from build123d import *

# Parameters (mm, degrees)
BOSS_EXTRUDE3_DEPTH     = 35
CUT_EXTRUDE4_START      = -33
CUT_EXTRUDE4_DEPTH      = 33
SHELL3_DEPTH            = 33
BOSS_EXTRUDE5_START     = 1
BOSS_EXTRUDE5_DEPTH     = 1
CUT_EXTRUDE5_DEPTH      = 88.114866699
CUT_EXTRUDE5_DEPTH_BACK = 88.114866699
SKETCH10_R              = 1.5
FILLET6_R               = 2
FILLET8_R               = 2
CUT_EXTRUDE7_REACH      = 151.75
SKETCH13_W              = 20
SKETCH13_H              = 20
CUT_EXTRUDE10_REACH     = 113.915
SKETCH16_W              = 19.05
SKETCH16_H              = 12.7
FILLET11_R              = 1


# Read off the part's stored shape, not the designer's step: Shell3
with BuildPart() as part:
    # Sketch4 → Boss-Extrude3 (new body)
    with BuildSketch(Plane(origin=(0, 0, 0), x_dir=(1, 0, 0), z_dir=(0, 1, 0))):
        with BuildLine():
            Line((-63, 40), (63, 40))
            ThreePointArc((63, 40), (67.949747468, 37.949747468), (70, 33))
            Line((70, 33), (70, -33))
            ThreePointArc((70, -33), (67.949747468, -37.949747468), (63, -40))
            Line((63, -40), (-63, -40))
            ThreePointArc((-63, -40), (-67.949747468, -37.949747468), (-70, -33))
            Line((-70, -33), (-70, 33))
            ThreePointArc((-70, 33), (-67.949747468, 37.949747468), (-63, 40))
        make_face()
    extrude(amount=BOSS_EXTRUDE3_DEPTH)

    # Sketch9 → Cut-Extrude4 (cut)
    with BuildSketch(Plane(origin=(0, 35, 0), x_dir=(1, 0, 0), z_dir=(0, 1, 0)).offset(CUT_EXTRUDE4_START)):
        with BuildLine():
            Line((-63, 26), (-70, 26))
            Line((-70, 26), (-70, 33))
            ThreePointArc((-70, 33), (-67.949747468, 37.949747468), (-63, 40))
            Line((-63, 40), (-56, 40))
            Line((-56, 40), (-56, 33))
            ThreePointArc((-56, 33), (-58.050252532, 28.050252532), (-63, 26))
        make_face()
        with BuildLine():
            Line((-63, -26), (-70, -26))
            Line((-70, -26), (-70, -33))
            ThreePointArc((-70, -33), (-67.949747468, -37.949747468), (-63, -40))
            Line((-63, -40), (-56, -40))
            Line((-56, -40), (-56, -33))
            ThreePointArc((-56, -33), (-58.050252532, -28.050252532), (-63, -26))
        make_face()
        with BuildLine():
            Line((56, -33), (56, -40))
            Line((56, -40), (63, -40))
            ThreePointArc((63, -40), (67.949747468, -37.949747468), (70, -33))
            Line((70, -33), (70, -26))
            Line((70, -26), (63, -26))
            ThreePointArc((63, -26), (58.050252532, -28.050252532), (56, -33))
        make_face()
        with BuildLine():
            Line((56, 33), (56, 40))
            Line((56, 40), (63, 40))
            ThreePointArc((63, 40), (67.949747468, 37.949747468), (70, 33))
            Line((70, 33), (70, 26))
            Line((70, 26), (63, 26))
            ThreePointArc((63, 26), (58.050252532, 28.050252532), (56, 33))
        make_face()
    extrude(amount=CUT_EXTRUDE4_DEPTH, mode=Mode.SUBTRACT)

    # Shell3 outline → Shell3 (cut)
    with BuildSketch(Plane(origin=(0, 0, 0), x_dir=(1, 0, 0), z_dir=(0, 1, 0))):
        with BuildLine():
            Line((-68, 24), (-68, -25.516685226))
            ThreePointArc((-68, -25.516685226), (-56.636038969, -26.636038969), (-55.516685226, -38))
            Line((-55.516685226, -38), (55.516685226, -38))
            ThreePointArc((55.516685226, -38), (56.636038969, -26.636038969), (68, -25.516685226))
            Line((68, -25.516685226), (68, 24))
            Line((68, 24), (63, 24))
            ThreePointArc((63, 24), (56.636038969, 26.636038969), (54, 33))
            Line((54, 33), (54, 38))
            Line((54, 38), (-54, 38))
            Line((-54, 38), (-54, 33))
            ThreePointArc((-54, 33), (-56.636038969, 26.636038969), (-63, 24))
            Line((-63, 24), (-68, 24))
        make_face()
    extrude(amount=SHELL3_DEPTH, mode=Mode.SUBTRACT)

    # Sketch11 → Boss-Extrude5 (add)
    with BuildSketch(Plane.XZ.offset(-1).offset(BOSS_EXTRUDE5_START)):
        with BuildLine():
            Line((68, 24), (63, 24))
            ThreePointArc((63, 24), (56.636038969, 26.636038969), (54, 33))
            Line((54, 33), (54, 38))
            Line((54, 38), (63, 38))
            ThreePointArc((63, 38), (66.535533906, 36.535533906), (68, 33))
            Line((68, 33), (68, 24))
        make_face()
        with BuildLine():
            Line((54, -33), (54, -38))
            Line((54, -38), (63, -38))
            ThreePointArc((63, -38), (66.535533906, -36.535533906), (68, -33))
            Line((68, -33), (68, -24))
            Line((68, -24), (63, -24))
            ThreePointArc((63, -24), (56.636038969, -26.636038969), (54, -33))
        make_face()
        with BuildLine():
            Line((-63, -24), (-68, -24))
            Line((-68, -24), (-68, -33))
            ThreePointArc((-68, -33), (-66.535533906, -36.535533906), (-63, -38))
            Line((-63, -38), (-54, -38))
            Line((-54, -38), (-54, -33))
            ThreePointArc((-54, -33), (-56.636038969, -26.636038969), (-63, -24))
        make_face()
        with BuildLine():
            Line((-54, 33), (-54, 38))
            Line((-54, 38), (-63, 38))
            ThreePointArc((-63, 38), (-66.535533906, 36.535533906), (-68, 33))
            Line((-68, 33), (-68, 24))
            Line((-68, 24), (-63, 24))
            ThreePointArc((-63, 24), (-56.636038969, 26.636038969), (-54, 33))
        make_face()
    extrude(amount=-BOSS_EXTRUDE5_DEPTH)

    # Sketch10 → Cut-Extrude5 (cut, two sides: drawn at the far end of the back side and taken through both)
    with BuildSketch(Plane(origin=(0, 2, 0), x_dir=(1, 0, 0), z_dir=(0, 1, 0)).offset(-CUT_EXTRUDE5_DEPTH_BACK)):
        with Locations(Location((-63, 33, 0), (0, 0, 270))):
            Circle(SKETCH10_R)
        with Locations(Location((63, 33, 0), (0, 0, 270))):
            Circle(SKETCH10_R)
        with Locations(Location((63, -33, 0), (0, 0, 270))):
            Circle(SKETCH10_R)
        with Locations(Location((-63, -33, 0), (0, 0, 270))):
            Circle(SKETCH10_R)
    extrude(amount=CUT_EXTRUDE5_DEPTH + CUT_EXTRUDE5_DEPTH_BACK, mode=Mode.SUBTRACT)

    # Fillet6
    fillet6_edges = [part.edges().sort_by_distance(p)[0] for p in [
        (68, 16.5, -24),
        (-54, 16.5, -38),
        (0, 33, -38),
        (-68, 33, 0.758342613),
        (0, 33, 38),
        (68, 33, 0.758342613),
        (-56.636038969, 33, 26.636038969),
        (-56.636038969, 33, -26.636038969),
        (-68, 16.5, -24),
        (-65.5, 33, -24),
        (-54, 33, -35.5),
        (56.636038969, 33, 26.636038969),
        (56.636038969, 33, -26.636038969),
        (54, 16.5, -38),
        (54, 33, -35.5),
        (65.5, 33, -24),
    ]]
    fillet(fillet6_edges, radius=FILLET6_R)

    # Fillet8
    fillet8_edges = [part.edges().sort_by_distance(p)[0] for p in [
        (0, 35, 40),
        (-58.050252532, 35, 28.050252532),
        (-66.5, 35, 26),
        (-56, 35, 36.5),
        (-58.050252532, 2, 28.050252532),
        (-56, 2, 36.5),
        (-66.5, 2, 26),
        (-70, 35, 0),
        (-58.050252532, 35, -28.050252532),
        (-56, 35, -36.5),
        (-66.5, 35, -26),
        (-58.050252532, 2, -28.050252532),
        (-66.5, 2, -26),
        (-56, 2, -36.5),
        (70, 35, 0),
        (58.050252532, 35, 28.050252532),
        (56, 35, 36.5),
        (66.5, 35, 26),
        (58.050252532, 2, 28.050252532),
        (66.5, 2, 26),
        (56, 2, 36.5),
        (0, 35, -40),
        (58.050252532, 35, -28.050252532),
        (66.5, 35, -26),
        (56, 35, -36.5),
        (58.050252532, 2, -28.050252532),
        (56, 2, -36.5),
        (66.5, 2, -26),
    ]]
    fillet(fillet8_edges, radius=FILLET8_R)

    # Sketch13 → Cut-Extrude7 (cut, up to next)
    with BuildSketch(Plane(origin=(70, 0, 0), x_dir=(0, 0, -1), z_dir=(1, 0, 0)), mode=Mode.PRIVATE) as cut_extrude7_sk1:
        with Locations((7.25040296, 18.065666935)):
            Rectangle(SKETCH13_W, SKETCH13_H)
    cut_extrude7_tool1 = extrude(cut_extrude7_sk1.sketch, amount=-CUT_EXTRUDE7_REACH, mode=Mode.PRIVATE) & part.part
    add(cut_extrude7_tool1.solids().sort_by_distance((70, 18.065667, -7.250403))[0], mode=Mode.SUBTRACT)

    # Sketch16 → Cut-Extrude10 (cut, up to next)
    with BuildSketch(Plane.XY.offset(40), mode=Mode.PRIVATE) as cut_extrude10_sk1:
        with Locations((-28.725, 14)):
            Rectangle(SKETCH16_W, SKETCH16_H)
    cut_extrude10_tool1 = extrude(cut_extrude10_sk1.sketch, amount=-CUT_EXTRUDE10_REACH, mode=Mode.PRIVATE) & part.part
    add(cut_extrude10_tool1.solids().sort_by_distance((-28.725, 14, 40))[0], mode=Mode.SUBTRACT)

    # Fillet11
    fillet11_edges = [part.edges().sort_by_distance(p)[0] for p in [
        (-19.2, 20.35, 39),
        (-19.2, 7.65, 39),
        (-38.25, 7.65, 39),
        (-38.25, 20.35, 39),
    ]]
    fillet(fillet11_edges, radius=FILLET11_R)


solid = part.part
Verification items for the finished model (mm, model axes). A direction names the side the tool comes from. Coordinates: 2 decimals unless noted, no trailing zeros. Order: outer loops, then holes, each group sorted by start corner. A loop starts at its lowest first (then second) coordinate and runs counter-clockwise, first axis right, second up. Notation, with made-up numbers: M 33.5,-18 L 49.5,-18 A27 ccw 49.5,9 Z; hole C -39,-10.5 d5. An arc over 180 degrees is marked long. Return JSON: item names as keys, results as strings.
1) Cross-section at A-A, the plane z = 14.5. Record the boundary of the cut face in (x, y).
Answer list:
{"outline": "M -70,0 L -68,0 L -68,31 A2 cw -66,33 L 66,33 A2 cw 68,31 L 68,0 L 70,0 L 70,33 A2 ccw 68,35 L -68,35 A2 ccw -70,33 Z"}
2) Gauge pin test, flat ends, axial feed: pin 1 (0.8 mm diameter, centred on x = -55, z = 35.5, fed in from +Y); pin 2 (7.5 mm diameter, centred on x = 65.5, y = 15.5, fed in from -Z); pin 3 (3.5 mm diameter, centred on y = 16.5, z = 36.5, fed in from -X); pin 4 (3.5 mm diameter, centred on x = -63, z = -33, fed in from -Y). Record the tip position at first contact, or that the pin passes through.
Answer list:
{"pin 1": "y = 34.91", "pin 2": "z = -26.11", "pin 3": "x = -56", "pin 4": "y = 0"}
3) Release check for a two-part mould opening along X. For faces 1 (the cylindrical face through (56.76, 15.283, 26.515)), 2 (the cylindrical face through (67.9, 1, -38)), 3 (the cylindrical face through (-58, 18.3, -28.1)), 4 (the flat face through (1, 16, 40)) record: +X half, -X half, draft (parallel to the pull), parting line (faces both ways), or undercut.
Answer list:
{"face 1": "undercut", "face 2": "+X half", "face 3": "-X half", "face 4": "draft"}
4) Thickness scan on L1, parallel to Z at x = 63, y = 0.7; L2, parallel to X at y = 7, z = -21.5; L3, parallel to Z at x = 15, y = 24.5. Record the ranges inside material, lowest first. Write a range as [from, to].
Answer list:
{"L1": "[-40, -34.5], [-31.5, -24], [24, 31.5], [34.5, 40]", "L2": "[-70, -68], [68, 70]", "L3": "[-40, -38], [38, 40]"}
5) Access from +Z, -Z, +X, -X, +Y, -Y to the whole of each face (thin tool, end or side, straight path). Record for faces 5 (the cylindrical face through (58.1, 18.3, 28)), 6 (the cylindrical face through (-56.566, 15.283, -26.706)), 7 (the cylindrical face through (-56.76, 15.283, 26.515)).
Answer list:
{"face 5": "+Z, +X, +Y", "face 6": "-Y", "face 7": "none"}
6) Cross-section at B-B, the plane x = 28. Record the boundary of the cut face in (y, z), and give its area (3 significant figures).
Answer list:
{"outline": "M 0,-40 L 33,-40 A2 ccw 35,-38 L 35,38 A2 ccw 33,40 L 0,40 L 0,38 L 31,38 A2 cw 33,36 L 33,-36 A2 cw 31,-38 L 0,-38 Z", "area": "292 mm2"}
